from build123d import *

# Parameters (mm, degrees)
F1_DEPTH = 3.2


with BuildPart() as f1:
    # F0 (on Top) → F1 (new body)
    with BuildSketch(Plane.XY):
        Polygon((-65.523831, 30), (-85.523831, 30), (-85.523831, 26.8), (-105.523831, 26.8), (-105.523831, 13.8), (-102.323831, 13.8), (-102.323831, -3.8), (-105.523831, -3.8), (-105.523831, -16.8), (-85.523831, -16.8), (-85.523831, -20), (-65.523831, -20), (-65.523831, -16.8), (-45.523831, -16.8), (-45.523831, -20), (-25.523831, -20), (-25.523831, -16.8), (-5.523831, -16.8), (-5.523831, -20), (14.476169, -20), (14.476169, -16.8), (34.476169, -16.8), (34.476169, -20), (54.476169, -20), (54.476169, -16.8), (74.476169, -16.8), (74.476169, -20), (94.476169, -20), (94.476169, -10), (91.276169, -10), (91.276169, 0), (94.476169, 0), (94.476169, 10), (91.276169, 10), (91.276169, 20), (94.476169, 20), (94.476169, 30), (74.476169, 30), (74.476169, 26.8), (54.476169, 26.8), (54.476169, 30), (34.476169, 30), (34.476169, 26.8), (14.476169, 26.8), (14.476169, 30), (-5.523831, 30), (-5.523831, 26.8), (-25.523831, 26.8), (-25.523831, 30), (-45.523831, 30), (-45.523831, 26.8), (-65.523831, 26.8), align=None)
    extrude(amount=F1_DEPTH)


solid = f1.part
Geometry check sheet. Reference: the model listing, model coordinates, mm. A direction names the side the tool comes from. Give positions to 0.01 mm unless a question says otherwise; leave off trailing zeros. Order: outer loops, then holes, each group sorted by start corner. A loop starts at its lowest first (then second) coordinate and runs counter-clockwise, first axis right, second up.
1) Material ranges on probe 1 along X at (y, z) = (27.5, 1.45); probe 2 along X at (y, z) = (16.5, 3.05); probe 3 along X at (y, z) = (6.5, 1), recorded low to high.
Results are:
probe 1: x = -85.52 to -65.52, -45.52 to -25.52, -5.52 to 14.48, 34.48 to 54.48, 74.48 to 94.48
probe 2: x = -105.52 to 91.28
probe 3: x = -102.32 to 94.48
2) Cross-section at A-A (y = -8). Record the boundary of the cut face in (x, z).
Results are:
outline: (-105.52, 0) - (91.28, 0) - (91.28, 3.2) - (-105.52, 3.2) - close
3) Gauge pin test, flat ends, axial feed: pin 1 (1.6 mm diameter, centred on x = -19, z = 1, fed in from -Y); pin 2 (1 mm diameter, centred on x = -93, z = 2, fed in from +Y); pin 3 (1.5 mm diameter, centred on y = 6.5, z = 1.5, fed in from -X). Record the tip position at first contact, or that the pin passes through.
Results are:
pin 1: stops at y = -16.8
pin 2: stops at y = 26.8
pin 3: stops at x = -102.32
4) Tool access check on faces 5 (the flat face through (-15, 26.8, 2)), 6 (the flat face through (-102.324, 5, 2)), 7 (the flat face through (24, -16.8, 2)), 8 (the flat face through (93, -10, 2)), 9 (the flat face through (-96, -16.8, 2)). Record the directions out of +Z, -Z, +X, -X, +Y, -Y that give a thin tool (end or side, any length) a straight path to the whole face; none if there is none.
Results are:
face 5: +Z, -Z, +Y
face 6: +Z, -Z, -X
face 7: +Z, -Z, -Y
face 8: +Z, -Z, +X
face 9: +Z, -Z, -X, -Y
5) Cross-section at B-B (x = 69.5). Record the boundary of the cut face in (y, z), then the cut area to 3 significant figures.
Results are:
outline: (-16.8, 0) - (26.8, 0) - (26.8, 3.2) - (-16.8, 3.2) - close
area: 140 mm2
6) Draft check along X on faces 1 (the flat face through (-105.524, 20, 2)), 2 (the flat face through (94.476, 25, 2)), 3 (the flat face through (-76, -20, 2)), 4 (the flat face through (-55, 26.8, 2)). Enter one of: released by +X, released by -X, zero draft, split by the parting line, or undercut.
Results are:
face 1: released by -X
face 2: released by +X
face 3: zero draft
face 4: undercut
